```python
from build123d import *

# Parameters (mm, degrees)
F0_R     = 0.75
F1_DEPTH = 3


with BuildPart() as f1:
    # F0 (on Front) → F1 (new body)
    with BuildSketch(Plane.XZ):
        Polygon((-100.5, -3), (-100.5, 0), (-80.5, 0), (-63.5, -17), (0, -17), (63.5, -17), (80.5, 0), (100.5, 0), (100.5, -3), (110.5, -3), (110.5, 0), (110.5, 3), (0, 3), (-110.5, 3), (-110.5, 0), (-110.5, -3), align=None)
        with Locations((-58.25, -15.25)):
            Circle(F0_R, mode=Mode.SUBTRACT)
        with Locations((58.25, -15.25)):
            Circle(F0_R, mode=Mode.SUBTRACT)
        Polygon((-62.257359, -14), (-76.257359, 0), (-62.257359, 0), align=None, mode=Mode.SUBTRACT)
        Polygon((-45.257359, 0), (-59.257359, -14), (-59.257359, 0), align=None, mode=Mode.SUBTRACT)
        Polygon((-55.014719, -14), (-41.014719, 0), (-27.014719, -14), align=None, mode=Mode.SUBTRACT)
        Polygon((-22.772078, -14), (-36.772078, 0), (-22.772078, 0), align=None, mode=Mode.SUBTRACT)
        Polygon((-5.772078, 0), (-19.772078, -14), (-19.772078, 0), align=None, mode=Mode.SUBTRACT)
        Polygon((-1.529437, 0), (-1.529437, -14), (-15.529437, -14), align=None, mode=Mode.SUBTRACT)
        Polygon((1.529437, -14), (1.529437, 0), (15.529437, -14), align=None, mode=Mode.SUBTRACT)
        Polygon((19.772078, 0), (19.772078, -14), (5.772078, 0), align=None, mode=Mode.SUBTRACT)
        Polygon((36.772078, 0), (22.772078, -14), (22.772078, 0), align=None, mode=Mode.SUBTRACT)
        Polygon((27.014719, -14), (41.014719, 0), (55.014719, -14), align=None, mode=Mode.SUBTRACT)
        Polygon((45.257359, 0), (59.257359, 0), (59.257359, -14), align=None, mode=Mode.SUBTRACT)
        Polygon((62.257359, -14), (62.257359, 0), (76.257359, 0), align=None, mode=Mode.SUBTRACT)
    extrude(amount=F1_DEPTH)


solid = f1.part
```
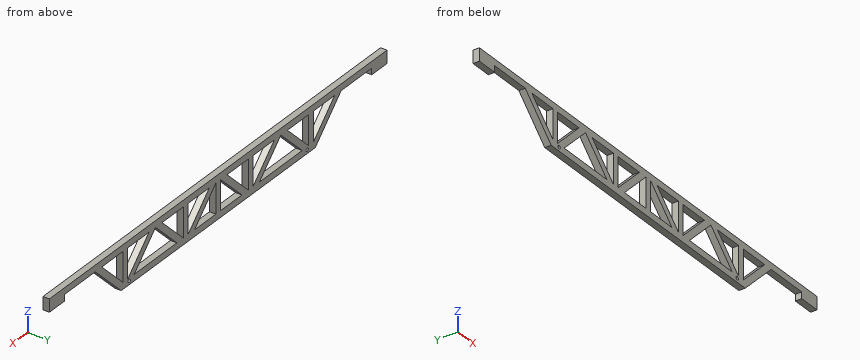
Check sheet for the modelled part. Datum: model origin and axes. Units: mm. Round coordinates to 2 decimals unless told otherwise and drop trailing zeros. Order: outer loops, then holes, each group sorted by start corner. A loop starts at its lowest first (then second) coordinate and runs counter-clockwise, first axis right, second up.
1) Go/stop test with flat-tipped pins: pin 1 Ø1.5 at (y, z) = (-1.5, -8) entering from +X; pin 2 Ø1.5 at (x, y) = (68.5, -1.5) entering from -Z; pin 3 Ø0.9 at (y, z) = (-1.5, -4.5) entering from -X. Record where each tip stops, or that it passes through.
2) Section check C-C (x = -52). Record the boundary of the cut face in (y, z).
3) Section check B-B (y = -1.45). Give the number of separate pieces and of enclosed holes in the cut face, and give its area (3 significant figures).
4) Section check A-A (x = 65.5). Record the boundary of the cut face in (y, z).
5) Scan lines: line 1 (Z direction, x = -58.25, y = -1.1); line 2 (Z direction, x = -27.5, y = -2); line 3 (Z direction, x = -83, y = -2.45). Record each from-to range of solid material in increasing order.
Result:
1. pin 1: stops at x = 73.25
1. pin 2: stops at z = -12.75
1. pin 3: stops at x = -76.45
2. outline: (-3, -17) - (0, -17) - (0, -14) - (-3, -14) - close; (-3, -10.99) - (0, -10.99) - (0, -6.74) - (-3, -6.74) - close; (-3, 0) - (0, 0) - (0, 3) - (-3, 3) - close
3. separate pieces: 1
3. enclosed holes: 14
3. area: 1,800 mm2
4. outline: (-3, -15) - (0, -15) - (0, -10.76) - (-3, -10.76) - close; (-3, 0) - (0, 0) - (0, 3) - (-3, 3) - close
5. line 1: z = -17 to -16, -14.5 to -12.99, 0 to 3
5. line 2: z = -17 to -14, -13.51 to -9.27, 0 to 3
5. line 3: z = 0 to 3
